```python
from build123d import *

# Parameters (mm, degrees)
F1_DEPTH = 300
F2_R     = 3.25
F3_DEPTH = 25
F5_DEPTH = 4
F8_DEPTH = 4


with BuildPart() as f1:
    # F0 (on Front) → F1 (new body)
    with BuildSketch(Plane.XZ):
        Polygon((0, 60), (0, 0), (80, 0), (80, 4), (4, 4), (4, 60), align=None)
    extrude(amount=F1_DEPTH)

    # F2 (on face) → F3 (cut)
    with BuildSketch(Plane.XY.offset(4)):
        with Locations((42, -20)):
            Circle(F2_R)
        with Locations((42, -280)):
            Circle(F2_R)
    extrude(amount=-F3_DEPTH, mode=Mode.SUBTRACT)

    # F4 (on Front) → F5 (join)
    with BuildSketch(Plane.XZ):
        Polygon((80, 4), (4, 60), (4, 4), align=None)
    extrude(amount=F5_DEPTH)

    # F7 (on offset) → F8 (join)
    with BuildSketch(Plane.XZ.offset(300)):
        Polygon((80, 4), (4, 60), (4, 4), align=None)
    extrude(amount=-F8_DEPTH)


solid = f1.part
```
Could you check a few things on this model? Use its own coordinates, in mm. A direction names the side the tool comes from. Give positions to 0.01 mm unless a question says otherwise; leave off trailing zeros. Order: outer loops, then holes, each group sorted by start corner. A loop starts at its lowest first (then second) coordinate and runs counter-clockwise, first axis right, second up.
Q1. Suppose I cut it at B-B, the plane y = -20. Write out the boundary of the cut face in (x, z), and give its area (3 significant figures).
Q2. We'd pull the mould along X, two halves only. Please class faces 3 (the cylindrical face through (43.5, -282.883, 2.028)), 4 (the flat face through (4, -148, 32)), 5 (the flat face through (31, 0, 24)), 6 (the cylindrical face through (45.1, -19.02, 2.03)): +X half, -X half, draft (parallel to the pull), parting line (faces both ways), or undercut.
Q3. If I drill on line 1 along Y through (x, z) = (42, 2.75); line 2 along Y through (x, z) = (16, 31); line 3 along X through (y, z) = (-280, 1), over which ranges is the centre line in solid material (lowest first)?
Q4. Suppose I cut it at D-D, the plane x = 19. Write out the boundary of the cut face in (y, z), and give its area (3 significant figures).
Q5. I'm going to push flat-ended pins straight in: P1, Ø3, axis at y = -116.5, z = 41, coming from the +X side; P2, Ø4, axis at x = 60.5, y = -75, coming from the +Z side. Where does each tip first touch, or does it pass through?
Q6. Suppose I cut it at C-C, the plane z = 55.5. Write out the boundary of the cut face in (x, y), and give its area (3 significant figures).
Q7. For faces 1 (the flat face through (42.53, -298.03, 31.61)), 2 (the flat face through (43, -148, 4)), which set-ups out of +Z, -Z, +X, -X, +Y, -Y let a thin tool reach every point of the face, with its end or its side?
Q8. Suppose I cut it at A-A, the plane x = 42. Write out the boundary of the cut face in (y, z).
Solution:
1. outline: (0, 0) - (38.75, 0) - (38.75, 4) - (4, 4) - (4, 60) - (0, 60) - close; (45.25, 0) - (80, 0) - (80, 4) - (45.25, 4) - close
1. area: 518 mm2
2. face 3: undercut
2. face 4: +X half
2. face 5: draft
2. face 6: undercut
3. line 1: y = -300 to -283.25, -276.75 to -23.25, -16.75 to 0
3. line 2: y = -300 to -296, -4 to 0
3. line 3: x = 0 to 38.75, 45.25 to 80
4. outline: (-300, 0) - (0, 0) - (0, 48.95) - (-4, 48.95) - (-4, 4) - (-296, 4) - (-296, 48.95) - (-300, 48.95) - close
4. area: 1,560 mm2
5. P1: stops at x = 4
5. P2: stops at z = 4
6. outline: (0, -300) - (10.11, -300) - (10.11, -296) - (4, -296) - (4, -4) - (10.11, -4) - (10.11, 0) - (0, 0) - close
6. area: 1,250 mm2
7. face 1: +Z, +X, +Y, -Y
7. face 2: +Z, +X
8. outline: (-300, 0) - (-283.25, 0) - (-283.25, 4) - (-296, 4) - (-296, 32) - (-300, 32) - close; (-276.75, 0) - (-23.25, 0) - (-23.25, 4) - (-276.75, 4) - close; (-16.75, 0) - (0, 0) - (0, 32) - (-4, 32) - (-4, 4) - (-16.75, 4) - close
